Part model, mm, in its own coordinate system. Round coordinates to 2 decimals unless told otherwise and drop trailing zeros. Write each loop counter-clockwise with the first axis right and the second up, starting at its lowest first coordinate (ties: lowest second). Pieces come first, ordered by that corner, then holes. Notation, with made-up numbers: (-2, 69) -> (42, 69) arc R27 ccw to (42, 106) -> close; hole circle Ø3 at (-14, 53). An arc over 180 degrees is marked (long way). Return JSON: item names as keys, results as strings. Group by question number.
(1) Saw through at A-A (y = -24). List the corners of the cut face in (x, z) (3 decimals).
(2) Saw through at C-C (x = 0). List the corners of the cut face in (y, z) (3 decimals).
(3) Drill centre lines: L1, parallel to Y at x = 0, z = 1.55; L2, parallel to X at y = -29, z = 0.9; L3, parallel to Y at x = -50.8, z = 2.1. Where is each one in solid material? Low to high. Write a range as from..to.
(4) Saw through at B-B (x = -90.5). List the corners of the cut face in (y, z) (3 decimals).
(5) Saw through at D-D (x = 50.8). List the corners of the cut face in (y, z) (3 decimals).
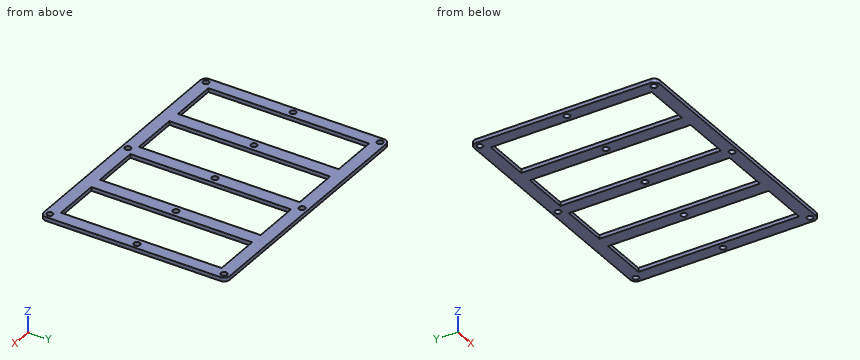
from build123d import *

# Parameters (mm, degrees)
SKETCH1_R           = 2.54
SKETCH1_W           = 39.624
SKETCH1_H           = 133.604
BOSS_EXTRUDE1_DEPTH = 3.175


with BuildPart() as part:
    # Sketch1 → Boss-Extrude1 (new body)
    with BuildSketch(Plane.XY):
        with BuildLine():
            Line((106.426, 24.765), (106.426, 72.39))
            ThreePointArc((106.426, 72.39), (105.012497326, 75.802497326), (101.6, 77.216))
            Line((101.6, 77.216), (-101.6, 77.216))
            ThreePointArc((-101.6, 77.216), (-105.012497326, 75.802497326), (-106.426, 72.39))
            Line((-106.426, 72.39), (-106.426, 24.765))
            Line((-106.426, 24.765), (-106.426, -24.765))
            Line((-106.426, -24.765), (-106.426, -72.39))
            ThreePointArc((-106.426, -72.39), (-105.012497326, -75.802497326), (-101.6, -77.216))
            Line((-101.6, -77.216), (101.6, -77.216))
            ThreePointArc((101.6, -77.216), (105.012497326, -75.802497326), (106.426, -72.39))
            Line((106.426, -72.39), (106.426, -24.765))
            Line((106.426, -24.765), (106.426, 24.765))
        make_face()
        with Locations((-101.6, -72.39)):
            Circle(SKETCH1_R, mode=Mode.SUBTRACT)
        with Locations((0, -72.39)):
            Circle(SKETCH1_R, mode=Mode.SUBTRACT)
        with Locations((25.4, 0)):
            Rectangle(SKETCH1_W, SKETCH1_H, mode=Mode.SUBTRACT)
        with Locations((101.6, -72.39)):
            Circle(SKETCH1_R, mode=Mode.SUBTRACT)
        with Locations((-101.6, 0)):
            Circle(SKETCH1_R, mode=Mode.SUBTRACT)
        with Locations((-76.2, 0)):
            Rectangle(SKETCH1_W, SKETCH1_H, mode=Mode.SUBTRACT)
        with Locations((-101.6, 72.39)):
            Circle(SKETCH1_R, mode=Mode.SUBTRACT)
        with Locations((-50.8, 0)):
            Circle(SKETCH1_R, mode=Mode.SUBTRACT)
        with Locations((-25.4, 0)):
            Rectangle(SKETCH1_W, SKETCH1_H, mode=Mode.SUBTRACT)
        Circle(SKETCH1_R, mode=Mode.SUBTRACT)
        with Locations((50.8, 0)):
            Circle(SKETCH1_R, mode=Mode.SUBTRACT)
        with Locations((0, 72.39)):
            Circle(SKETCH1_R, mode=Mode.SUBTRACT)
        with Locations((76.2, 0)):
            Rectangle(SKETCH1_W, SKETCH1_H, mode=Mode.SUBTRACT)
        with Locations((101.6, 0)):
            Circle(SKETCH1_R, mode=Mode.SUBTRACT)
        with Locations((101.6, 72.39)):
            Circle(SKETCH1_R, mode=Mode.SUBTRACT)
    extrude(amount=BOSS_EXTRUDE1_DEPTH)


solid = part.part
Computed values:
{
 "1": {"outline": "(-106.426, 0) -> (-96.012, 0) -> (-96.012, 3.175) -> (-106.426, 3.175) -> close; (-56.388, 0) -> (-45.212, 0) -> (-45.212, 3.175) -> (-56.388, 3.175) -> close; (-5.588, 0) -> (5.588, 0) -> (5.588, 3.175) -> (-5.588, 3.175) -> close; (45.212, 0) -> (56.388, 0) -> (56.388, 3.175) -> (45.212, 3.175) -> close; (96.012, 0) -> (106.426, 0) -> (106.426, 3.175) -> (96.012, 3.175) -> close"},
 "2": {"outline": "(-77.216, 0) -> (-74.93, 0) -> (-74.93, 3.175) -> (-77.216, 3.175) -> close; (-69.85, 0) -> (-2.54, 0) -> (-2.54, 3.175) -> (-69.85, 3.175) -> close; (2.54, 0) -> (69.85, 0) -> (69.85, 3.175) -> (2.54, 3.175) -> close; (74.93, 0) -> (77.216, 0) -> (77.216, 3.175) -> (74.93, 3.175) -> close"},
 "3": {"L1": "-77.22..-74.93, -69.85..-2.54, 2.54..69.85, 74.93..77.22", "L2": "-106.43..-96.01, -56.39..-45.21, -5.59..5.59, 45.21..56.39, 96.01..106.43", "L3": "-77.22..-2.54, 2.54..77.22"},
 "4": {"outline": "(-77.216, 0) -> (-66.802, 0) -> (-66.802, 3.175) -> (-77.216, 3.175) -> close; (66.802, 0) -> (77.216, 0) -> (77.216, 3.175) -> (66.802, 3.175) -> close"},
 "5": {"outline": "(-77.216, 0) -> (-2.54, 0) -> (-2.54, 3.175) -> (-77.216, 3.175) -> close; (2.54, 0) -> (77.216, 0) -> (77.216, 3.175) -> (2.54, 3.175) -> close"}
}
